from build123d import *

# Parameters (mm, degrees)
SKETCH1_W           = 1.8
SKETCH1_H           = 21.5
SKETCH1_H_2         = 5.625
SKETCH1_W_2         = 2.1
SKETCH1_H_3         = 7.75
SKETCH1_H_4         = 8.125
BOSS_EXTRUDE1_DEPTH = 1.25
FILLET1_R           = 0.5
BOSS_EXTRUDE2_DEPTH = 2
SKETCH4_W           = 1.8
SKETCH4_H           = 0.1
BOSS_EXTRUDE3_DEPTH = 8.125


with BuildPart() as part:
    # Sketch1 → Boss-Extrude1 (new body, symmetric)
    with BuildSketch(Plane(origin=(0, 0, 0), x_dir=(1, 0, 0), z_dir=(0, 1, 0))):
        Rectangle(SKETCH1_W, SKETCH1_H)
        Polygon((-2.4375, 10.75), (-0.9, 10.75), (0.9, 10.75), (2.4375, 10.75), (2.4375, 12.55), (-2.4375, 12.55), align=None)
        with Locations((0, 7.9375)):
            Rectangle(SKETCH1_W, SKETCH1_H_2)
        with Locations((-1.95, 1.25)):
            Rectangle(SKETCH1_W_2, SKETCH1_H_3)
        with Locations((1.95, 1.25)):
            Rectangle(SKETCH1_W_2, SKETCH1_H_3)
        with Locations((0, -6.6875)):
            Rectangle(SKETCH1_W, SKETCH1_H_4)
    extrude(amount=BOSS_EXTRUDE1_DEPTH, both=True)

    # Fillet1
    fillet1_edges = [part.edges().sort_by_distance(p)[0] for p in [
        (-1.95, 1.25, -5.125),
        (-3, 1.25, -1.25),
        (-1.95, 1.25, 2.625),
        (-0.9, 1.25, 6.6875),
        (0, 1.25, 10.75),
        (0.9, 1.25, 6.6875),
        (1.95, 1.25, 2.625),
        (3, 1.25, -1.25),
        (-0.9, 1.25, -7.9375),
        (1.95, 1.25, -5.125),
        (0.9, 1.25, -7.9375),
        (1.66875, 1.25, -10.75),
        (2.4375, 1.25, -11.65),
        (0, 1.25, -12.55),
        (-2.4375, 1.25, -11.65),
        (-1.66875, 1.25, -10.75),
    ]]
    fillet(fillet1_edges, radius=FILLET1_R)

    # Sketch3 → Boss-Extrude2 (add)
    with BuildSketch(Plane.XY.offset(2.625)):
        with BuildLine():
            ThreePointArc((2.90473751, 0.75), (0, 3), (-2.90473751, 0.75))
            Line((-2.90473751, 0.75), (-0.9, 0.75))
            Line((-0.9, 0.75), (0.9, 0.75))
            Line((0.9, 0.75), (2.90473751, 0.75))
        make_face()
        with BuildLine():
            Line((2.727178029, -1.25), (0.9, -1.25))
            Line((0.9, -1.25), (-0.9, -1.25))
            Line((-0.9, -1.25), (-2.727178029, -1.25))
            ThreePointArc((-2.727178029, -1.25), (0, -3), (2.727178029, -1.25))
        make_face()
    extrude(amount=-BOSS_EXTRUDE2_DEPTH)

    # Sketch4 → Boss-Extrude3 (add)
    with BuildSketch(Plane.XY.offset(2.625)):
        with BuildLine():
            ThreePointArc((2.679085665, 1.35), (0, 3), (-2.679085665, 1.35))
            Line((-2.679085665, 1.35), (-0.9, 1.35))
            Line((-0.9, 1.35), (0.9, 1.35))
            Line((0.9, 1.35), (2.679085665, 1.35))
        make_face()
        with BuildLine():
            Line((0.9, -1.35), (-0.9, -1.35))
            Line((-0.9, -1.35), (-2.679085665, -1.35))
            ThreePointArc((-2.679085665, -1.35), (0, -3), (2.679085665, -1.35))
            Line((2.679085665, -1.35), (0.9, -1.35))
        make_face()
        with BuildLine():
            Line((0.9, -1.25), (-0.9, -1.25))
            Line((-0.9, -1.25), (-0.9, 0.75))
            ThreePointArc((-0.9, 0.75), (-0.753553391, 1.103553391), (-0.4, 1.25))
            Line((-0.4, 1.25), (0.4, 1.25))
            ThreePointArc((0.4, 1.25), (0.753553391, 1.103553391), (0.9, 0.75))
            Line((0.9, 0.75), (0.9, -1.25))
        make_face()
        with BuildLine():
            Line((0.9, 1.35), (-0.9, 1.35))
            Line((-0.9, 1.35), (-0.9, 0.75))
            ThreePointArc((-0.9, 0.75), (-0.753553391, 1.103553391), (-0.4, 1.25))
            Line((-0.4, 1.25), (0.4, 1.25))
            ThreePointArc((0.4, 1.25), (0.753553391, 1.103553391), (0.9, 0.75))
            Line((0.9, 0.75), (0.9, 1.35))
        make_face()
        with Locations((0, -1.3)):
            Rectangle(SKETCH4_W, SKETCH4_H)
    extrude(amount=BOSS_EXTRUDE3_DEPTH)

    # Sketch5 one side → Revolve1 (revolve)
    with BuildSketch(Plane(origin=(0, 0, 0), x_dir=(0, 0, -1), z_dir=(1, 0, 0))):
        with BuildLine():
            Line((12.55, -0.25), (13.2, -0.25))
            ThreePointArc((13.2, -0.25), (13.009619408, 0.209619408), (12.55, 0.4))
            Line((12.55, 0.4), (12.55, -0.25))
        make_face()
    revolve(axis=Axis((0, -0.25, -12.55), (0, 0, -1)))


solid = part.part
Geometry check sheet. Reference: the model listing, model coordinates, mm. A direction names the side the tool comes from. Coordinates: 2 decimals unless noted, no trailing zeros. Order: outer loops, then holes, each group sorted by start corner. A loop starts at its lowest first (then second) coordinate and runs counter-clockwise, first axis right, second up. Notation, with made-up numbers: M 72.5,18.25 L 116.5,18.25 A26 cw 116.5,54.25 Z; hole C -11,-3.75 d7. An arc over 180 degrees is marked long. Use CSV: the item, a comma, the result in double quotes.
Item 1: Cross-section at A-A on z = 9. Record the cut outline in (x, y), then the cut area to 3 significant figures.
Returned:
outline,"M -2.68,-1.35 A3 ccw 2.68,-1.35 L 0.9,-1.35 L 0.9,1.35 L 2.68,1.35 A3 ccw -2.68,1.35 L -0.9,1.35 L -0.9,-1.35 Z"
area,"17.5 mm2"
Item 2: Tool access check on faces 1 (the flat face through (-0.9, 0, -8)), 2 (the flat face through (2.438, 0, -12)), 3 (the flat face through (2, 1.35, 7)), 4 (the flat face through (-2.438, 0, -12)), 5 (the flat face through (-2, -1.35, 7)). Record the directions out of +Z, -Z, +X, -X, +Y, -Y that give a thin tool (end or side, any length) a straight path to the whole face; none if there is none.
Returned:
face 1,"-X, +Y, -Y"
face 2,"-Z, +X, +Y, -Y"
face 3,"+Z, +X"
face 4,"-Z, -X, +Y, -Y"
face 5,"+Z, -X"
Item 3: Gauge pin test, flat ends, axial feed: pin 1 Ø0.9 at (x, y) = (-1, 2) entering from -Z (3 decimals); pin 2 Ø1 at (y, z) = (-0.5, -6.5) entering from -X; pin 3 Ø2 at (x, z) = (2, 4.5) entering from +Y; pin 4 Ø1 at (y, z) = (-2, -2) entering from -X. Record the tip position at first contact, or that the pin passes through.
Returned:
pin 1,"stops at z = 0.625"
pin 2,"stops at x = -0.9"
pin 3,"stops at y = 2.83"
pin 4,"passes through"
Item 4: Cross-section at C-C on z = -7.5. Record the cut outline in (x, y).
Returned:
outline,"M -0.9,-1.25 L 0.9,-1.25 L 0.9,0.75 A0.5 ccw 0.4,1.25 L -0.4,1.25 A0.5 ccw -0.9,0.75 Z"
Item 5: Cross-section at B-B on y = -1.75. Record the cut outline in (x, z) (3 decimals).
Returned:
outline,"M -2.437,0.625 L 2.437,0.625 L 2.437,10.75 L -2.437,10.75 Z"
Item 6: Mould release check, pull along Z, two halves, no side actions. Record for faces 6 (the flat face through (0.9, 0, -8)), 7 (the flat face through (0.9, 0, 7)), 8 (the flat face through (2, 0, 2.625)): pulls with the +Z half, pulls with the -Z half, needs draft (parallel to the pull), parting line crosses it, or undercut.
Returned:
face 6,"undercut"
face 7,"needs draft"
face 8,"pulls with the +Z half"
Item 7: Thickness scan on line 1 along Z through (x, y) = (1.5, -0.5) (3 decimals); line 2 along Y through (x, z) = (-1.75, 8.5); line 3 along Z through (x, y) = (1.5, 1.75) (3 decimals). Record the ranges inside material, lowest first.
Returned:
line 1,"z = -12.55 to -10.75, -5.125 to 2.625"
line 2,"y = -2.44 to -1.35, 1.35 to 2.44"
line 3,"z = 0.625 to 10.75"
